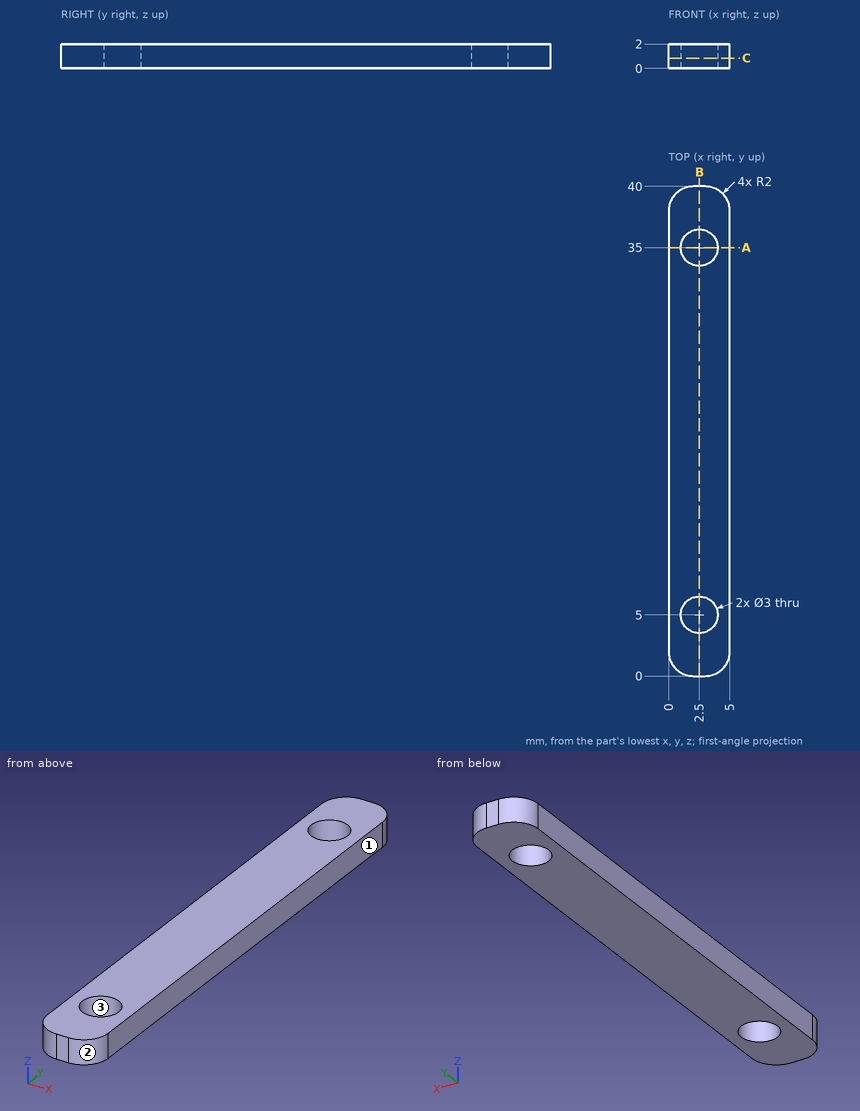
Answer from the drawing. Dimensions are ordinates in mm from the lowest x, y and z of the part. Round coordinates to 2 decimals unless told otherwise and drop trailing zeros. Order: outer loops, then holes, each group sorted by start corner. A loop starts at its lowest first (then second) coordinate and runs counter-clockwise, first axis right, second up. Notation, with made-up numbers: (-34.5, 86) - (-21.5, 86) arc R24 ccw to (-21.5, 111) - close; hole circle Ø9 at (77.25, -31). An arc over 180 degrees is marked (long way). Put each result on its own line as item: value. Start each with the question number.
(1) Given P1, Ø1.8, axis at x = 2.5, y = 35, coming from the -Z side, flat-ended and moving along its own axis, determine where the tip first touches the part or whether it passes through.
(2) Determine the mould class of the marked faces 1, 2 and 3 for opening direction Y: released by +Y, released by -Y, zero draft, split by the parting line, or undercut.
(3) Find section C-C (z = 0.85). Give the vertices of the cut face in (x, y), plus the area to 3 significant figures.
(4) Find section B-B (x = 2.5). Give the vertices of the cut face in (y, z).
(5) Straight lines are drawn through the part: probe 1 along Y at (x, z) = (2.5, 0.75); probe 2 along Y at (x, z) = (1.3, 1.65); probe 3 along X at (y, z) = (35, 1.3). For each, find the intervals that lie inside material, in ascending order. Write a range as from..to.
(6) Find section A-A (y = 35). Give the vertices of the cut face in (x, z), plus the area to 3 significant figures.
Reply:
1. P1: through
2. face 1: zero draft
2. face 2: released by -Y
2. face 3: undercut
3. outline: (0, 2) arc R2 ccw to (2, 0) - (3, 0) arc R2 ccw to (5, 2) - (5, 38) arc R2 ccw to (3, 40) - (2, 40) arc R2 ccw to (0, 38) - close; hole circle Ø3 at (2.5, 5); hole circle Ø3 at (2.5, 35)
3. area: 182 mm^2
4. outline: (0, 0) - (3.5, 0) - (3.5, 2) - (0, 2) - close; (6.5, 0) - (33.5, 0) - (33.5, 2) - (6.5, 2) - close; (36.5, 0) - (40, 0) - (40, 2) - (36.5, 2) - close
5. probe 1: 0..3.5, 6.5..33.5, 36.5..40
5. probe 2: 0.13..4.1, 5.9..34.1, 35.9..39.87
5. probe 3: 0..1, 4..5
6. outline: (0, 0) - (1, 0) - (1, 2) - (0, 2) - close; (4, 0) - (5, 0) - (5, 2) - (4, 2) - close
6. area: 4.00 mm^2
